Could you check a few things on this model? Use its own coordinates, in mm. Round coordinates to 2 decimals unless told otherwise and drop trailing zeros. Loops run counter-clockwise (first coordinate to the right, second up) from the corner with the lowest first, then second, coordinate; pieces in that order, holes last.
from build123d import *

# Parameters (mm, degrees)
F0_R     = 11.05
F1_DEPTH = 7
F2_SIZE  = 3.5
F3_SIZE  = 3.49999


# Not quite as in the source:
# - a fillet or chamfer is up to 0.001 mm smaller than in the source, because OpenCascade refuses the exact size


with BuildPart() as f1:
    # F0 (on Top) → F1 (new body)
    with BuildSketch(Plane.XY):
        Polygon((0, 45), (-15, 15), (0, 15), align=None)
        Polygon((0, 45), (0, 15), (15, 15), align=None)
        Polygon((0, 15), (-15, 15), (-15, 0), (-15, -15), (0, -15), (15, -15), (15, 0), (15, 15), align=None)
        Circle(F0_R, mode=Mode.SUBTRACT)
        Polygon((-15, -15), (-15, 0), (-45, 0), align=None)
        Polygon((-15, 0), (-15, 15), (-45, 0), align=None)
        Polygon((0, -15), (-15, -15), (0, -45), align=None)
        Polygon((15, -15), (0, -15), (0, -45), align=None)
        Polygon((45, 0), (15, 0), (15, -15), align=None)
        Polygon((45, 0), (15, 15), (15, 0), align=None)
    extrude(amount=F1_DEPTH)

    # F2
    f2_edges = [f1.edges().sort_by_distance(p)[0] for p in [
        (30, -7.5, 7),
        (7.5, -30, 7),
        (-7.5, -30, 7),
        (-30, -7.5, 7),
        (-30, 7.5, 7),
        (-7.5, 30, 7),
        (7.5, 30, 7),
        (30, 7.5, 7),
    ]]
    chamfer(f2_edges, length=F2_SIZE)

    # F3 (size 3.5 in the source; OpenCascade refuses exactly that, so slightly less here)
    f3_edges = [f1.edges().sort_by_distance(p)[0] for p in [
        (30, 7.5, 0),
        (7.5, 30, 0),
        (-7.5, 30, 0),
        (-30, 7.5, 0),
        (-30, -7.5, 0),
        (-7.5, -30, 0),
        (7.5, -30, 0),
        (30, -7.5, 0),
    ]]
    chamfer(f3_edges, length=F3_SIZE)


solid = f1.part
Item 1: We'd pull the mould along X, two halves only. Please class faces 1 (the flat face through (-28.467, 6.282, 5.274)), 2 (the flat face through (-11.2, 0.2, 0)), 3 (the cylindrical face through (-2.395, -10.787, 3.451)), 4 (the flat face through (6.07, -28.9, 5.27)): released by +X, released by -X, zero draft, split by the parting line, or undercut.
Results list:
face 1: released by -X
face 2: zero draft
face 3: undercut
face 4: released by +X
Item 2: If I drill on line 1 along Y through (x, z) = (19, 5.25); line 2 along Y through (x, z) = (-6.5, 6.5); line 3 along Y through (x, z) = (3, 2.75), over which ranges is the centre line in solid material (lowest first)?
Results list:
line 1: y = -11.04 to 11.04
line 2: y = -25.29 to -8.94, 8.94 to 25.29
line 3: y = -37.32 to -10.63, 10.63 to 37.32
Item 3: Will these pins go through, and if not, where does the flat tip stop? pin 1 (1 mm diameter, centred on x = 12.5, z = 3.5, fed in from +Y); pin 2 (1.5 mm diameter, centred on y = 22.5, z = 2.5, fed in from -X); pin 3 (10 mm diameter, centred on x = -22, y = -9.5, fed in from -Z); pin 4 (3 mm diameter, centred on x = 30.5, z = 1.5, fed in from -Y).
Results list:
pin 1: stops at y = 21
pin 2: stops at x = -11.05
pin 3: stops at z = 0
pin 4: stops at y = -6.85
Item 4: If we section it at B-B, the plane z = 4.75: Please give me the cut outline in (x, y).
Results list:
outline: (-42.2, 0) - (-14.07, -14.07) - (0, -42.2) - (14.07, -14.07) - (42.2, 0) - (14.07, 14.07) - (0, 42.2) - (-14.07, 14.07) - close; hole circle Ø22.1 at (0, 0)
